from build123d import *

# Parameters (mm, degrees)
SKETCH_1_W                  = 116
SKETCH_1_H                  = 14
EXTRUDE_763_DEPTH           = 2
CUT_EXTRUDE_1069_DEPTH      = 2
SKETCH_5_W                  = 19
SKETCH_5_H                  = 35
SKETCH_5_W_2                = 20
SKETCH_5_H_2                = 30
CUT_EXTRUDE_1759_DEPTH      = 2
EXTRUDE_3355_DEPTH          = 12
SKETCH_7_W                  = 2
SKETCH_7_H                  = 2
EXTRUDE_4350_DEPTH          = 12
SKETCH_2_R                  = 2
SKETCH_2_R_2                = 1.5
CUT_EXTRUDE_5250_DEPTH      = 12
CUT_EXTRUDE_5250_DEPTH_BACK = 2


with BuildPart() as part:
    # 草图1 → Extrude 763 (new body)
    with BuildSketch(Plane(origin=(0, 0, 0), x_dir=(1, 0, 0), z_dir=(0, 1, 0))):
        with BuildLine():
            Line((-60, -29.5), (-60, -80))
            ThreePointArc((-60, -80), (0, -100), (60, -80))
            Line((60, -80), (60, -29.5))
            Line((60, -29.5), (58, -29.5))
            Line((58, -29.5), (-58, -29.5))
            Line((-58, -29.5), (-60, -29.5))
        make_face()
        with Locations((0, -22.5)):
            Rectangle(SKETCH_1_W, SKETCH_1_H)
    extrude(amount=EXTRUDE_763_DEPTH)

    # 草图3 → Cut-Extrude 1069 (cut)
    with BuildSketch(Plane(origin=(0, 2, 0), x_dir=(1, 0, 0), z_dir=(0, 1, 0))):
        Polygon((-40, -15.5), (40, -15.5), (32.5, -29.5), (-32.5, -29.5), align=None)
    extrude(amount=-CUT_EXTRUDE_1069_DEPTH, mode=Mode.SUBTRACT)

    # 草图5 → Cut-Extrude 1759 (cut)
    with BuildSketch(Plane(origin=(0, 2, 0), x_dir=(1, 0, 0), z_dir=(0, 1, 0))):
        with Locations((-25.5, -52)):
            Rectangle(SKETCH_5_W, SKETCH_5_H)
        with Locations((25.5, -52)):
            Rectangle(SKETCH_5_W, SKETCH_5_H)
        with Locations((0, -52)):
            Rectangle(SKETCH_5_W_2, SKETCH_5_H_2)
    extrude(amount=-CUT_EXTRUDE_1759_DEPTH, mode=Mode.SUBTRACT)

    # 草图6 → Extrude 3355 (add)
    with BuildSketch(Plane(origin=(0, 2, 0), x_dir=(1, 0, 0), z_dir=(0, 1, 0))):
        with BuildLine():
            Line((-58, -81.461647418), (-58, -29.5))
            Line((-58, -29.5), (-60, -29.5))
            Line((-60, -29.5), (-60, -80))
            ThreePointArc((-60, -80), (-59.004526125, -80.737016893), (-58, -81.461647418))
        make_face()
        with BuildLine():
            Line((60, -29.5), (58, -29.5))
            Line((58, -29.5), (58, -81.461647418))
            ThreePointArc((58, -81.461647418), (59.004526125, -80.737016893), (60, -80))
            Line((60, -80), (60, -29.5))
        make_face()
        Polygon((-37, -32.5), (-37, -69.5), (-35, -69.5), (-35, -34.5), (-16, -34.5), (-16, -69.5), (-14, -69.5), (-14, -32.5), align=None)
        Polygon((35, -69.5), (37, -69.5), (37, -32.5), (14, -32.5), (14, -69.5), (16, -69.5), (16, -34.5), (35, -34.5), align=None)
    extrude(amount=EXTRUDE_3355_DEPTH)

    # 草图7 → Extrude 4350 (add)
    with BuildSketch(Plane(origin=(0, 2, 0), x_dir=(1, 0, 0), z_dir=(0, 1, 0))):
        with Locations((-57, -30.5)):
            Rectangle(SKETCH_7_W, SKETCH_7_H)
        Polygon((-32.5, -29.5), (-58, -29.5), (-58, -15.5), (-40, -15.5), align=None)
        with Locations((57, -30.5)):
            Rectangle(SKETCH_7_W, SKETCH_7_H)
        Polygon((32.5, -29.5), (58, -29.5), (58, -15.5), (40, -15.5), align=None)
    extrude(amount=EXTRUDE_4350_DEPTH)

    # 草图2 → Cut-Extrude 5250 (cut, two sides)
    with BuildSketch(Plane(origin=(0, 2, 0), x_dir=(1, 0, 0), z_dir=(0, 1, 0))) as cut_extrude_5250_sk:
        with Locations((-45, -22)):
            Circle(SKETCH_2_R)
        with Locations((-40, -82)):
            Circle(SKETCH_2_R)
        with Locations((40, -82)):
            Circle(SKETCH_2_R)
        with Locations((45, -22)):
            Circle(SKETCH_2_R)
        with Locations((-50, -35.5)):
            Circle(SKETCH_2_R_2)
        with Locations((-50, -68.5)):
            Circle(SKETCH_2_R_2)
        with Locations((50, -68.5)):
            Circle(SKETCH_2_R_2)
        with Locations((50, -35.5)):
            Circle(SKETCH_2_R_2)
    extrude(amount=CUT_EXTRUDE_5250_DEPTH, mode=Mode.SUBTRACT)
    extrude(cut_extrude_5250_sk.sketch, amount=-CUT_EXTRUDE_5250_DEPTH_BACK, mode=Mode.SUBTRACT)


solid = part.part
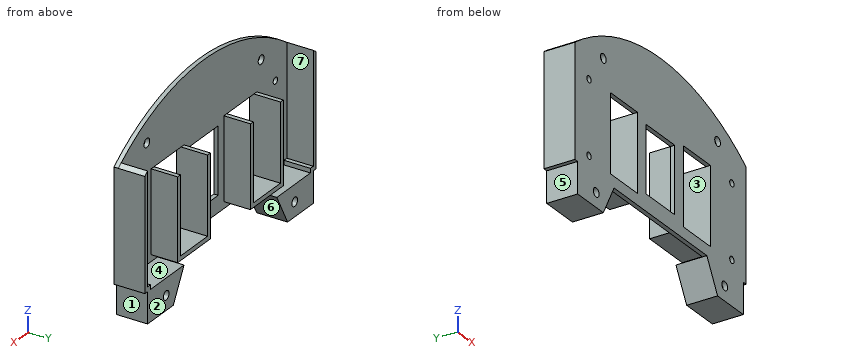
Model file for the job. Use its own axes, mm. Face numbers are marked on the shaded views. A direction names the side the tool comes from. Coordinates: 2 decimals unless noted, no trailing zeros. Order: outer loops, then holes, each group sorted by start corner. A loop starts at its lowest first (then second) coordinate and runs counter-clockwise, first axis right, second up. Notation, with made-up numbers: M 41.25,-16 L 76.25,-16 A32 cw 76.25,14 Z; hole C 37.5,8 d2. An arc over 180 degrees is marked long. Return JSON: item names as keys, results as strings.
1. Saw through at B-B (x = -20). Give the cut face in (y, z), and give its area (3 significant figures).
Ans:
{"outline": "M 0,29.5 L 2,29.5 L 2,32.5 L 14,32.5 L 14,34.5 L 0,34.5 Z; M 0,69.5 L 2,69.5 L 2,97.98 L 0,97.98 Z", "area": "91.0 mm^2"}
2. Tool access for the marked faces 4, 5, 6 and 7: list every direction of +Z, -Z, +X, -X, +Y, -Y with a clear straight run to the whole face (end or side of a thin tool).
Ans:
{"face 4": "+Y", "face 5": "-Z, -X, +Y, -Y", "face 6": "-Z, +Y, -Y", "face 7": "+Z, +Y"}
3. Saw through at D-D (x = -50). Give the cut face in (y, z).
Ans:
{"outline": "M 0,15.5 L 14,15.5 L 14,29.5 L 2,29.5 L 2,34 L 0,34 Z; M 0,37 L 2,37 L 2,67 L 0,67 Z; M 0,70 L 2,70 L 2,86.6 L 0,86.6 Z"}
4. Flat gauge pins, fed straight in: pin 1 (0.6 mm diameter, centred on x = -23.5, y = 0.5, fed in from -Z); pin 2 (6.5 mm diameter, centred on x = 40, z = 82, fed in from +Y); pin 3 (1 mm diameter, centred on x = 35, y = 3.5, fed in from +Z); pin 4 (4 mm diameter, centred on x = -3, z = 79.5, fed in from -Y). Where does each tip first touch, or does it go through?
Ans:
{"pin 1": "z = 29.5", "pin 2": "y = 2", "pin 3": "z = 69.5", "pin 4": "y = 0"}
5. Pull direction X, two halves, no side cores. Call the marked faces 1, 2 and 3: +X half, -X half, draft (parallel to the pull), parting line (faces both ways), or undercut.
Ans:
{"face 1": "+X half", "face 2": "draft", "face 3": "undercut"}
6. Saw through at C-C (y = 5.75). Give the number of separate pieces and of enclosed holes in the cut face, and give its area (3 significant figures).
Ans:
{"separate pieces": "4", "enclosed holes": "2", "area": "1,170 mm^2"}
7. Saw through at A-A (z = 43). Give the cut face in (x, y), and give its area (3 significant figures).
Ans:
{"outline": "M -60,0 L -35,0 L -35,14 L -37,14 L -37,2 L -58,2 L -58,14 L -60,14 Z; M -16,0 L -10,0 L -10,2 L -14,2 L -14,14 L -16,14 Z; M 10,0 L 16,0 L 16,14 L 14,14 L 14,2 L 10,2 Z; M 35,0 L 60,0 L 60,14 L 58,14 L 58,2 L 37,2 L 37,14 L 35,14 Z", "area": "268 mm^2"}
8. Drill centre lines: probe 1 along X at (y, z) = (3.75, 36); probe 2 along X at (y, z) = (1.05, 68.5); probe 3 along X at (y, z) = (0.5, 52). Where is each one in solid material? Low to high.
Ans:
{"probe 1": "-60 to -58, -37 to -35, -16 to -14, 14 to 16, 35 to 37, 58 to 60", "probe 2": "-60 to -51.5, -48.5 to -35, -16 to 16, 35 to 48.5, 51.5 to 60", "probe 3": "-60 to -35, -16 to -10, 10 to 16, 35 to 60"}
